Read the model definition and answer for the solid it produces. Units are mm, in the model's axes. Face numbers are marked on the shaded views. A direction names the side the tool comes from. Coordinates: 2 decimals unless noted, no trailing zeros. Loops run counter-clockwise (first coordinate to the right, second up) from the corner with the lowest first, then second, coordinate; pieces in that order, holes last.
Q1. Which of the six approach directions +Z, -Z, +X, -X, +Y, -Y give full straight-line access (tool end or side, diameter ignored) to the marked faces 1, 2, 3 and 4?
Q2. Straight lines are drawn through the part: line 1 (X direction, y = 28, z = 23); line 2 (Z direction, x = 0, y = 28.5); line 3 (X direction, y = 33, z = 17.5). For each, find the intervals that lie inside material, in ascending order.
Q3. Section D-D (y = 14) is taken. Give the vertices of the cut face in (x, z), then the cut area to 3 significant figures.
Q4. Section C-C (z = 30) is taken. Give the vertices of the cut face in (x, y).
Q5. Section A-A (x = -39) is taken. Give the vertices of the cut face in (y, z), then the cut area to 3 significant figures.
Q6. Flat-ended cylindrical pins translate along their axes: P1, Ø2, axis at x = -36.5, z = 35, coming from the +Y side; P2, Ø8, axis at y = 17, z = 32.5, coming from the +X side; P3, Ø4, axis at x = 30.5, z = 24, coming from the -Y side. Find the tip coordinate at first contact, or state that the pin passes through.
Q7. Section B-B (y = 26) is taken. Give the vertices of the cut face in (x, z).
Q8. The mould has two halves that part along Z. Classify the marked faces 5, 6 and 7: pulls with the +Z half, pulls with the -Z half, needs draft (parallel to the pull), parting line crosses it, or undercut.
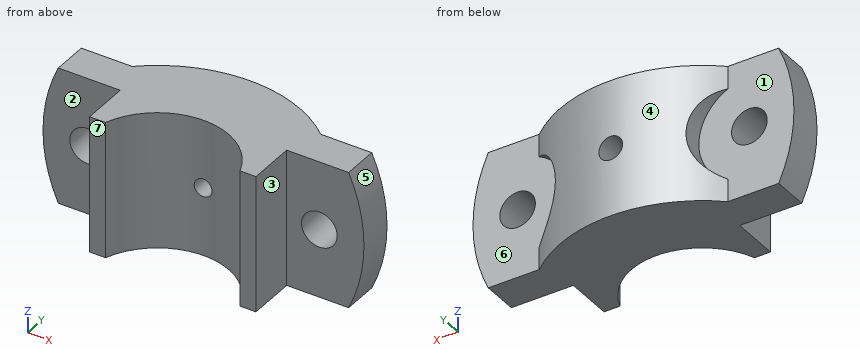
from build123d import *

# Parameters (mm, degrees)
BOSS_EXTRUDE1_DEPTH  = 46
CUT_EXTRUDE1_START   = -4.166957121
CUT_EXTRUDE1_DEPTH   = 17.166957121
CUT_EXTRUDE1_START_2 = 18
CUT_EXTRUDE1_2_DEPTH = 10
SKETCH4_R            = 3
CUT_EXTRUDE2_DEPTH   = 77.26270392
SKETCH5_R            = 17
CUT_EXTRUDE3_DEPTH   = 77.262703957
SKETCH6_R            = 6
CUT_EXTRUDE4_DEPTH   = 77.262703957
CUT_EXTRUDE5_DEPTH   = 86.650452531


with BuildPart() as part:
    # Sketch1 → Boss-Extrude1 (new body)
    with BuildSketch(Plane.XY):
        with BuildLine():
            Line((-28, 8), (-22.627416998, 8))
            ThreePointArc((-22.627416998, 8), (0, 24), (22.627416998, 8))
            Line((22.627416998, 8), (28, 8))
            Line((28, 8), (28, 24))
            Line((28, 24), (54, 24))
            Line((54, 24), (54, 36))
            Line((54, 36), (31.749015733, 36))
            ThreePointArc((31.749015733, 36), (0, 48), (-31.749015733, 36))
            Line((-31.749015733, 36), (-54, 36))
            Line((-54, 36), (-54, 24))
            Line((-54, 24), (-28, 24))
            Line((-28, 24), (-28, 8))
        make_face()
    extrude(amount=BOSS_EXTRUDE1_DEPTH)

    # Cut-Extrude1: read off the stored shape, not the designer's step
    # Cut-Extrude1 outline → Cut-Extrude1 (cut)
    with BuildSketch(Plane(origin=(0, 36, 0), x_dir=(1, 0, 0), z_dir=(0, 1, 0)).offset(CUT_EXTRUDE1_START)):
        with BuildLine():
            add(Edge.make_bspline(
                [(0, -19), (-1.057527997, -19), (-2.091087742, -19.434088276), (-3.566323367, -20.909614388), (-3.999433765, -21.953884044), (-4.00056506, -24.04178128), (-3.576219278, -25.07994956), (-2.083227921, -26.574310552), (-1.045821073, -26.9996204), (1.042915307, -27.000379072), (2.087446575, -26.567981834), (3.563947107, -25.094327717), (3.998968512, -24.060310778), (4.001027689, -21.947486084), (3.568016054, -20.912331491), (2.093312914, -19.435292521), (1.057527997, -19), (0, -19)],
                knots=[0, 0, 0, 0, 0.125, 0.125, 0.25, 0.25, 0.375, 0.375, 0.5, 0.5, 0.625, 0.625, 0.75, 0.75, 0.875, 0.875, 1, 1, 1, 1], degree=3))
        make_face()
    extrude(amount=CUT_EXTRUDE1_DEPTH, mode=Mode.SUBTRACT)

    # Cut-Extrude1 2 outline → Cut-Extrude1 2 (add)
    with BuildSketch(Plane.XY.offset(CUT_EXTRUDE1_START_2)):
        with BuildLine():
            ThreePointArc((4.00000004, 31.83304297), (-2.3e-08, 32), (-4.000000085, 31.833042966))
            Line((-4.000000085, 31.833042966), (4.00000004, 31.83304297))
        make_face()
    extrude(amount=CUT_EXTRUDE1_2_DEPTH)

    # Sketch4 → Cut-Extrude2 (cut, through all)
    with BuildSketch(Plane(origin=(0, 36, 0), x_dir=(1, 0, 0), z_dir=(0, 1, 0))):
        with Locations(Location((0, -23, 0), (0, 0, 270))):
            Circle(SKETCH4_R)
    extrude(amount=-CUT_EXTRUDE2_DEPTH, mode=Mode.SUBTRACT)

    # Sketch5 → Cut-Extrude3 (cut, through all)
    with BuildSketch(Plane(origin=(0, 36, 0), x_dir=(1, 0, 0), z_dir=(0, 1, 0))):
        with Locations((-39, -23)):
            Circle(SKETCH5_R)
        with Locations((39, -23)):
            Circle(SKETCH5_R)
    extrude(amount=CUT_EXTRUDE3_DEPTH, mode=Mode.SUBTRACT)

    # Sketch6 → Cut-Extrude4 (cut, through all)
    with BuildSketch(Plane(origin=(0, 36, 0), x_dir=(1, 0, 0), z_dir=(0, 1, 0))):
        with Locations(Location((-39, -23, 0), (0, 0, 270))):
            Circle(SKETCH6_R)
        with Locations(Location((39, -23, 0), (0, 0, 270))):
            Circle(SKETCH6_R)
    extrude(amount=-CUT_EXTRUDE4_DEPTH, mode=Mode.SUBTRACT)

    # Sketch8 → Cut-Extrude5 (cut, through all)
    with BuildSketch(Plane(origin=(0, 0, 0), x_dir=(1, 0, 0), z_dir=(0, 1, 0))):
        with BuildLine():
            Line((-48.61841215, -46.5), (-63.61841215, -46.5))
            Line((-63.61841215, -46.5), (-63.61841215, 0.5))
            Line((-63.61841215, 0.5), (-48.61841215, 0.5))
            ThreePointArc((-48.61841215, 0.5), (-54, -23), (-48.61841215, -46.5))
        make_face()
    cut_extrude5 = extrude(amount=CUT_EXTRUDE5_DEPTH, mode=Mode.SUBTRACT)

    # Mirror1: Cut-Extrude5 across plane
    add(cut_extrude5.mirror(Plane(origin=(0, 0, 0), x_dir=(0, 0, 1), z_dir=(1, 0, 0))), mode=Mode.SUBTRACT)


solid = part.part
Numbers:
1. face 1: -X, +Y
1. face 2: +Z, -Z, -X, -Y
1. face 3: +Z, -Z, +X, -Y
1. face 4: +Z, -Z, +Y
2. line 1: x = -54 to -45, -33 to -3, 3 to 33, 45 to 54
2. line 2: z = 0 to 20, 26 to 46
2. line 3: x = -53.72 to -41.4, -36.6 to 36.6, 41.4 to 53.72
3. outline: (-28, 0) - (-19.49, 0) - (-19.49, 46) - (-28, 46) - close; (19.49, 0) - (28, 0) - (28, 46) - (19.49, 46) - close
3. area: 783 mm2
4. outline: (-53.54, 24) - (-28, 24) - (-28, 8) - (-22.63, 8) arc R24 cw to (22.63, 8) - (28, 8) - (28, 24) - (53.54, 24) - (53.54, 36) - (23.51, 36) - (23.51, 41.85) arc R48 ccw to (-23.51, 41.85) - (-23.51, 36) - (-53.54, 36) - close
5. outline: (24, 0) - (36, 0) - (36, 17) - (24, 17) - close; (24, 29) - (36, 29) - (36, 46) - (24, 46) - close
5. area: 408 mm2
6. P1: stops at y = 36
6. P2: stops at x = 28
6. P3: stops at y = 24
7. outline: (-48.86, 0) - (48.86, 0) arc R54 ccw to (48.86, 46) - (-48.86, 46) arc R54 ccw to start; hole circle Ø12 at (-39, 23); hole circle Ø6 at (0, 23); hole circle Ø12 at (39, 23)
8. face 5: parting line crosses it
8. face 6: undercut
8. face 7: needs draft
